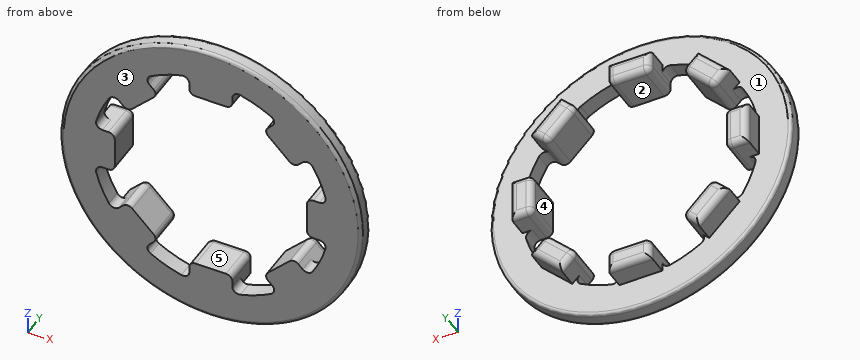
```python
from build123d import *

# Parameters (mm, degrees)
SKETCH2_R                = 4.725
SKETCH2_R_2              = 3.715
BOSS_EXTRUDE1_DEPTH      = 0.5
SKETCH3_W                = 1.35
SKETCH3_H                = 0.7
BOSS_EXTRUDE2_DEPTH      = 1.25
FILLET1_R                = 0.2
CIRPATTERN1_COUNT        = 8
FILLET1_OF_CIRPATTERN1_R = 0.2
FILLET2_R                = 0.1


with BuildPart() as part:
    # Sketch2 → Boss-Extrude1 (new body)
    with BuildSketch(Plane(origin=(0, 0, 0), x_dir=(1, 0, 0), z_dir=(0, 1, 0))):
        with Locations(Location((0, 0, 0), (0, 0, 270))):
            Circle(SKETCH2_R)
        with Locations(Location((0, 0, 0), (0, 0, 270))):
            Circle(SKETCH2_R_2, mode=Mode.SUBTRACT)
    extrude(amount=BOSS_EXTRUDE1_DEPTH)

    # Sketch3 → Boss-Extrude2 (add)
    with BuildSketch(Plane.XZ):
        with Locations((0, -3.365)):
            Rectangle(SKETCH3_W, SKETCH3_H)
    boss_extrude2 = extrude(amount=-BOSS_EXTRUDE2_DEPTH)

    # Fillet1
    fillet1_edges = [part.edges().sort_by_distance(p)[0] for p in [
        (-0.675, 0.25, -3.653163013),
        (0.675, 0.25, -3.653163013),
        (0.675, 1.25, -3.365),
        (0.675, 0.625, -3.015),
        (0, 1.25, -3.715),
        (-0.675, 1.25, -3.365),
        (0, 1.25, -3.015),
        (-0.675, 0.625, -3.015),
    ]]
    fillet(fillet1_edges, radius=FILLET1_R)

    # CirPattern1: Boss-Extrude2 ×8 about axis
    cirpattern1_axis = Axis((0, 0, 0), (0, 1, 0))
    for i in range(1, CIRPATTERN1_COUNT):
        add(boss_extrude2.rotate(cirpattern1_axis, i * 360 / CIRPATTERN1_COUNT))

    # Fillet1 of CirPattern1
    fillet1_of_cirpattern1_edges = [part.edges().sort_by_distance(p)[0] for p in [
        (-3.060473417, 0.25, -2.105879262),
        (-2.105879262, 0.25, -3.060473417),
        (-1.902117241, 1.25, -2.856711396),
        (-1.654629868, 0.625, -2.609224023),
        (-2.626901692, 1.25, -2.626901692),
        (-2.856711396, 1.25, -1.902117241),
        (-2.131926945, 1.25, -2.131926945),
        (-2.609224023, 0.625, -1.654629868),
        (-3.653163013, 0.25, 0.675),
        (-3.653163013, 0.25, -0.675),
        (-3.365, 1.25, -0.675),
        (-3.015, 0.625, -0.675),
        (-3.715, 1.25, 0),
        (-3.365, 1.25, 0.675),
        (-3.015, 1.25, 0),
        (-3.015, 0.625, 0.675),
        (-2.105879262, 0.25, 3.060473417),
        (-3.060473417, 0.25, 2.105879262),
        (-2.856711396, 1.25, 1.902117241),
        (-2.609224023, 0.625, 1.654629868),
        (-2.626901692, 1.25, 2.626901692),
        (-1.902117241, 1.25, 2.856711396),
        (-2.131926945, 1.25, 2.131926945),
        (-1.654629868, 0.625, 2.609224023),
        (0.675, 0.25, 3.653163013),
        (-0.675, 0.25, 3.653163013),
        (-0.675, 1.25, 3.365),
        (-0.675, 0.625, 3.015),
        (0, 1.25, 3.715),
        (0.675, 1.25, 3.365),
        (0, 1.25, 3.015),
        (0.675, 0.625, 3.015),
        (3.060473417, 0.25, 2.105879262),
        (2.105879262, 0.25, 3.060473417),
        (1.902117241, 1.25, 2.856711396),
        (1.654629868, 0.625, 2.609224023),
        (2.626901692, 1.25, 2.626901692),
        (2.856711396, 1.25, 1.902117241),
        (2.131926945, 1.25, 2.131926945),
        (2.609224023, 0.625, 1.654629868),
        (3.653163013, 0.25, -0.675),
        (3.653163013, 0.25, 0.675),
        (3.365, 1.25, 0.675),
        (3.015, 0.625, 0.675),
        (3.715, 1.25, 0),
        (3.365, 1.25, -0.675),
        (3.015, 1.25, 0),
        (3.015, 0.625, -0.675),
        (2.105879262, 0.25, -3.060473417),
        (3.060473417, 0.25, -2.105879262),
        (2.856711396, 1.25, -1.902117241),
        (2.609224023, 0.625, -1.654629868),
        (2.626901692, 1.25, -2.626901692),
        (1.902117241, 1.25, -2.856711396),
        (2.131926945, 1.25, -2.131926945),
        (1.654629868, 0.625, -2.609224023),
    ]]
    fillet(fillet1_of_cirpattern1_edges, radius=FILLET1_OF_CIRPATTERN1_R)

    # Fillet2
    fillet2_edges = [part.edges().sort_by_distance(p)[0] for p in [
        (0, 0, -4.725),
        (0, 0.5, -4.725),
    ]]
    fillet(fillet2_edges, radius=FILLET2_R)


solid = part.part
```
For this review, take the finished solid that the model builds, in its own axes (mm). Face numbers are marked on the shaded views. A direction names the side the tool comes from. Give positions to 0.01 mm unless a question says otherwise; leave off trailing zeros. Write each loop counter-clockwise with the first axis right and the second up, starting at its lowest first coordinate (ties: lowest second). Pieces come first, ordered by that corner, then holes. Notation, with made-up numbers: M 46,9.25 L 92,9.25 A31 ccw 92,39.25 Z; hole C 32,4.25 d8. An arc over 180 degrees is marked long. Answer as a JSON object with one key per item and string values. Group by question number.
Item 1: For pin 1 Ø0.6 at (x, y) = (3.5, 0.5) entering from +Z; pin 2 Ø0.5 at (y, z) = (1, 0) entering from -X (3 decimals); pin 3 Ø0.6 at (y, z) = (0.5, -3.5) entering from -X, all flat-tipped, find the tip position at first contact; note any pin that passes through.
Item 2: For probe 1 along X at (y, z) = (0.85, -0.5) (3 decimals); probe 2 along Z at (x, y) = (-3.5, 1.05) (3 decimals); probe 3 along Y at (x, z) = (-2.5, 2.5), list the stretches that pass through material, from the lowest coordinate up. Write a range as [from, to].
Item 3: Draft analysis for pull direction X (two halves, no side actions). For the marked faces 3, 4 and 5, state which applies: +X half, -X half, draft (parallel to the pull), parting line (faces both ways), or undercut.
Item 4: Tool access review of the marked faces 1 and 2: name each direction out of +Z, -Z, +X, -X, +Y, -Y from which nothing blocks a thin tool from reaching the whole face with its end or side.
Item 5: Consider section B-B on y = 0.65. Count the separate pieces of the cut face and the enclosed holes in it, plus the area to 3 significant figures.
Item 6: Consider section A-A on z = 0. Write out the cut boundary in (x, y) (3 decimals), plus the area to 3 significant figures.
Check result:
{
 "1": {"pin 1": "stops at z = 3.46", "pin 2": "stops at x = -3.715", "pin 3": "stops at x = -3.46"},
 "2": {"probe 1": "x = [-3.715, -3.017], [3.017, 3.715]", "probe 2": "z = [-0.675, 0.675]", "probe 3": "y = [0, 1.25]"},
 "3": {"face 3": "draft", "face 4": "undercut", "face 5": "undercut"},
 "4": {"face 1": "+Y", "face 2": "+Y, -Y"},
 "5": {"separate pieces": "8", "enclosed holes": "0", "area": "7.42 mm^2"},
 "6": {"outline": "M -4.725,0.1 A0.1 ccw -4.625,0 L -3.015,0 L -3.015,1.05 A0.2 ccw -3.215,1.25 L -3.515,1.25 A0.2 ccw -3.715,1.05 L -3.715,0.5 L -4.625,0.5 A0.1 ccw -4.725,0.4 Z; M 3.015,0 L 4.625,0 A0.1 ccw 4.725,0.1 L 4.725,0.4 A0.1 ccw 4.625,0.5 L 3.715,0.5 L 3.715,1.05 A0.2 ccw 3.515,1.25 L 3.215,1.25 A0.2 ccw 3.015,1.05 Z", "area": "2.72 mm^2"}
}
